Study the drawing (mm; zero at the part's minimum x, y, z) and answer. A direction names the side the tool comes from. Give positions to 0.01 mm unless a question says otherwise; leave off trailing zeros. Write each loop counter-clockwise with the first axis right and the second up, starting at its lowest first coordinate (ties: lowest second). Pieces come first, ordered by that corner, then holes.
1) Straight lines are drawn through the part: probe 1 along X at (y, z) = (356, 715); probe 2 along Y at (x, z) = (804, 663.5); probe 3 along Z at (x, y) = (511.5, 243.5). For each, find the intervals that lie inside material, in ascending order.
2) Given pin 1 Ø10 at (x, y) = (806, 722) entering from +Z; pin 2 Ø3 at (x, y) = (798, 146.5) entering from -Z, each flat-ended and moving along its own axis, determine where each tip first touches the part or whether it passes through.
3) Find section B-B (z = 412). Determine the outline of the cut face in (x, y), plus the area to 3 significant figures.
4) Find section C-C (x = 65.5). Determine the outline of the cut face in (y, z), plus the area to 3 significant figures.
5) Find section A-A (y = 92). Determine the outline of the cut face in (x, z).
6) A tool of negligible diameter and unlimited length cuts with its end or side. For the marked faces 1, 2 and 3, from which of +Z, -Z, +X, -X, +Y, -Y can it reach the whole face along a straight path? Write none if from no direction.
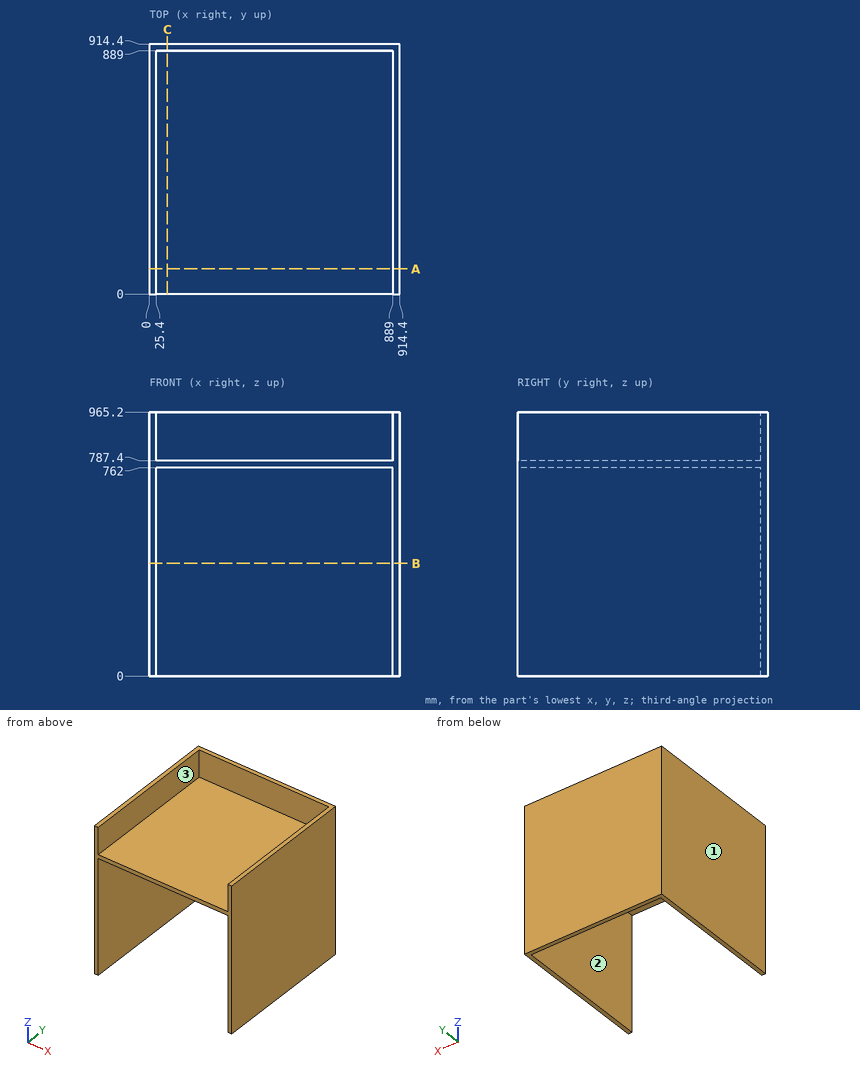
Results:
1. probe 1: x = 0 to 25.4, 889 to 914.4
1. probe 2: y = 889 to 914.4
1. probe 3: z = 762 to 787.4
2. pin 1: stops at z = 787.4
2. pin 2: stops at z = 762
3. outline: (0, 0) - (25.4, 0) - (25.4, 889) - (889, 889) - (889, 0) - (914.4, 0) - (914.4, 914.4) - (0, 914.4) - close
3. area: 68,400 mm2
4. outline: (0, 762) - (889, 762) - (889, 0) - (914.4, 0) - (914.4, 965.2) - (889, 965.2) - (889, 787.4) - (0, 787.4) - close
4. area: 47,100 mm2
5. outline: (0, 0) - (25.4, 0) - (25.4, 762) - (889, 762) - (889, 0) - (914.4, 0) - (914.4, 965.2) - (889, 965.2) - (889, 787.4) - (25.4, 787.4) - (25.4, 965.2) - (0, 965.2) - close
6. face 1: +Z, -Z, -X, +Y, -Y
6. face 2: -Z, -Y
6. face 3: +Z, -Y
